Read the model definition and answer for the solid it produces. Units are mm, in the model's axes. Round coordinates to 2 decimals unless told otherwise and drop trailing zeros. Write each loop counter-clockwise with the first axis right and the second up, starting at its lowest first coordinate (ties: lowest second). Pieces come first, ordered by that corner, then holes.
from build123d import *

# Parameters (mm, degrees)
F0_W     = 50.8
F0_H     = 101.6
F0_R     = 7.62
F1_DEPTH = 12.7
F2_R     = 5.08


with BuildPart() as f1:
    # F0 (on Front) → F1 (new body, symmetric)
    with BuildSketch(Plane.XZ):
        Rectangle(F0_W, F0_H)
        with Locations((0, -29.069694)):
            Circle(F0_R, mode=Mode.SUBTRACT)
        with Locations((0, 29.069694)):
            Circle(F0_R, mode=Mode.SUBTRACT)
    extrude(amount=F1_DEPTH, both=True)

    # F2
    f2_edges = [f1.edges().sort_by_distance(p)[0] for p in [
        (25.4, 0, 50.8),
        (-25.4, 0, 50.8),
        (25.4, 0, -50.8),
        (-25.4, 0, -50.8),
    ]]
    fillet(f2_edges, radius=F2_R)


solid = f1.part
Q1. Section C-C (y = -8.75) is taken. Determine the outline of the cut face in (x, z), then the cut area to 3 significant figures.
Verdict:
outline: (-25.4, -45.72) arc R5.08 ccw to (-20.32, -50.8) - (20.32, -50.8) arc R5.08 ccw to (25.4, -45.72) - (25.4, 45.72) arc R5.08 ccw to (20.32, 50.8) - (-20.32, 50.8) arc R5.08 ccw to (-25.4, 45.72) - close; hole circle Ø15.24 at (0, -29.07); hole circle Ø15.24 at (0, 29.07)
area: 4,770 mm2
Q2. Determine the mould class of faces 1 (the cylindrical face through (-0.992, 0.178, 36.625)), 2 (the cylindrical face through (23.951, -0.178, -49.272)), 3 (the flat face through (0, 12.7, 1)), 4 (the cylindrical face through (23.951, 0.178, 49.272)) for opening direction Z: pulls with the +Z half, pulls with the -Z half, needs draft (parallel to the pull), parting line crosses it, or undercut.
Verdict:
face 1: undercut
face 2: pulls with the -Z half
face 3: needs draft
face 4: pulls with the +Z half
Q3. Section A-A (x = 0) is taken. Determine the outline of the cut face in (y, z).
Verdict:
outline: (-12.7, -50.8) - (12.7, -50.8) - (12.7, -36.69) - (-12.7, -36.69) - close; (-12.7, -21.45) - (12.7, -21.45) - (12.7, 21.45) - (-12.7, 21.45) - close; (-12.7, 36.69) - (12.7, 36.69) - (12.7, 50.8) - (-12.7, 50.8) - close
Q4. Section B-B (z = -28) is taken. Determine the outline of the cut face in (x, y).
Verdict:
outline: (-25.4, -12.7) - (-7.54, -12.7) - (-7.54, 12.7) - (-25.4, 12.7) - close; (7.54, -12.7) - (25.4, -12.7) - (25.4, 12.7) - (7.54, 12.7) - close
Q5. Straight lines are drawn through the part: probe 1 along Z at (x, y) = (0, 2); probe 2 along Z at (x, y) = (6.5, 11.5); probe 3 along X at (y, z) = (-9, -29.5). For each, find the intervals that lie inside material, in ascending order.
Verdict:
probe 1: z = -50.8 to -36.69, -21.45 to 21.45, 36.69 to 50.8
probe 2: z = -50.8 to -33.05, -25.09 to 25.09, 33.05 to 50.8
probe 3: x = -25.4 to -7.61, 7.61 to 25.4
